Model file for the job. Use its own axes, mm. Give positions to 0.01 mm unless a question says otherwise; leave off trailing zeros. Loops run counter-clockwise (first coordinate to the right, second up) from the corner with the lowest first, then second, coordinate; pieces in that order, holes last. Notation, with made-up numbers: M 10,-29 L 40,-29 A27 ccw 40,-8 Z; hole C -14,20.5 d3. An arc over 180 degrees is marked long. Answer in a Markdown table with one row per item.
```python
from build123d import *

# Parameters (mm, degrees)
F0_W     = 210
F0_H     = 110
F1_DEPTH = 80
F3_DEPTH = 80
F4_R     = 10


with BuildPart() as f1:
    # F0 (on Top) → F1 (new body)
    with BuildSketch(Plane.XY):
        with Locations((32.656658, -16.551609)):
            Rectangle(F0_W, F0_H)
    extrude(amount=F1_DEPTH)

    # F2 (on face) → F3 (cut)
    with BuildSketch(Plane.XY.offset(80)):
        with BuildLine():
            Line((7.656658, -71.551609), (57.656658, -71.551609))
            ThreePointArc((57.656658, -71.551609), (32.656658, -46.398145), (7.656658, -71.551609))
        make_face()
    extrude(amount=-F3_DEPTH, mode=Mode.SUBTRACT)

    # F4
    f4_edges = [f1.edges().sort_by_distance(p)[0] for p in [
        (-72.343342, 38.448391, 40),
        (137.656658, 38.448391, 40),
    ]]
    fillet(f4_edges, radius=F4_R)


solid = f1.part
```
(1) Flat gauge pin, fed straight in: P1, Ø12, axis at x = 107.5, y = 16, coming from the -Z side. Where does the tip first touch, or does it go through?
Established:
| item | result |
|---|---|
| P1 | stops at z = 0 |
(2) Wall check: L1, parallel to X at y = -50, z = 19.5; L2, parallel to X at y = -52, z = 36; L3, parallel to Y at x = 16.5, z = 32. Give the ranges that are in metal, low to high.
Established:
| item | result |
|---|---|
| L1 | x = -72.34 to 19.73, 45.58 to 137.66 |
| L2 | x = -72.34 to 16.89, 48.43 to 137.66 |
| L3 | y = -52.32 to 38.45 |
(3) Mould opens along X. For faces 1 (the cylindrical face through (33.209, -46.404, 40.56)), 2 (the cylindrical face through (-69.492, 35.441, 40.56)), 3 (the cylindrical face through (134.65, 35.597, 40.56)) say: pulls with the +X half, pulls with the -X half, needs draft (parallel to the pull), parting line crosses it, or undercut.
Established:
| item | result |
|---|---|
| face 1 | undercut |
| face 2 | pulls with the -X half |
| face 3 | pulls with the +X half |
(4) Saw through at B-B, the plane y = -60.5. Give the cut face in (x, z), and give its area (3 significant figures).
Established:
| item | result |
|---|---|
| outline | M -72.34,0 L 10.16,0 L 10.16,80 L -72.34,80 Z; M 55.16,0 L 137.66,0 L 137.66,80 L 55.16,80 Z |
| area | 13,200 mm2 |
(5) Saw through at A-A, the plane z = 70.5. Give the cut face in (x, y), and give its area (3 significant figures).
Established:
| item | result |
|---|---|
| outline | M -72.34,-71.55 L 7.66,-71.55 A25 cw long 57.66,-71.55 L 137.66,-71.55 L 137.66,28.45 A10 ccw 127.66,38.45 L -62.34,38.45 A10 ccw -72.34,28.45 Z |
| area | 22,100 mm2 |
(6) Saw through at C-C, the plane x = 37. Give the cut face in (y, z), and give its area (3 significant figures).
Established:
| item | result |
|---|---|
| outline | M -46.78,0 L 38.45,0 L 38.45,80 L -46.78,80 Z |
| area | 6,820 mm2 |
